from build123d import *

# Parameters (mm, degrees)
BOSS_EXTRUDE1_DEPTH = 60
FILLET1_R           = 5
SKETCH2_R           = 5
CUT_EXTRUDE1_DEPTH  = 75
SKETCH3_W           = 5
SKETCH3_H           = 60
BOSS_EXTRUDE2_DEPTH = 15
FILLET3_R           = 3


with BuildPart() as part:
    # Sketch1 → Boss-Extrude1 (new body)
    with BuildSketch(Plane.XY):
        Polygon((0, 0), (35, 0), (35, -20), (0, -20), (0, -25), (40, -25), (40, 5), (0, 5), align=None)
    extrude(amount=BOSS_EXTRUDE1_DEPTH)

    # Fillet1
    fillet1_edges = [part.edges().sort_by_distance(p)[0] for p in [
        (35, -20, 30),
        (35, 0, 30),
    ]]
    fillet(fillet1_edges, radius=FILLET1_R)

    # Sketch2 → Cut-Extrude1 (cut)
    with BuildSketch(Plane(origin=(0, 5, 0), x_dir=(1, 0, 0), z_dir=(0, 1, 0))):
        with Locations(Location((15, -44, 0), (0, 0, 180))):
            Circle(SKETCH2_R)
        with Locations(Location((15, -16, 0), (0, 0, 270))):
            Circle(SKETCH2_R)
    extrude(amount=-CUT_EXTRUDE1_DEPTH, mode=Mode.SUBTRACT)

    # Sketch3 → Boss-Extrude2 (add)
    with BuildSketch(Plane.XZ.offset(25)):
        with Locations((35, 30)):
            Rectangle(SKETCH3_W, SKETCH3_H)
    extrude(amount=BOSS_EXTRUDE2_DEPTH)

    # Fillet3
    fillet3_edges = [part.edges().sort_by_distance(p)[0] for p in [
        (35, -40, 0),
        (35, -40, 60),
    ]]
    fillet(fillet3_edges, radius=FILLET3_R)


solid = part.part
Build history of the part. All positions in model axes, mm. A direction names the side the tool comes from. Round coordinates to 2 decimals unless told otherwise and drop trailing zeros. Write each loop counter-clockwise with the first axis right and the second up, starting at its lowest first coordinate (ties: lowest second). Pieces come first, ordered by that corner, then holes. Notation, with made-up numbers: M -15,3.5 L 8,3.5 A13 cw 8,9.5 Z; hole C -6.75,45.25 d5. An arc over 180 degrees is marked long. Use CSV: the item, a comma, the result in double quotes.
1. Saw through at A-A (x = 15). Give the cut face in (y, z).
Reply:
outline,"M -25,0 L -20,0 L -20,11 L -25,11 Z; M -25,21 L -20,21 L -20,39 L -25,39 Z; M -25,49 L -20,49 L -20,60 L -25,60 Z; M 0,0 L 5,0 L 5,11 L 0,11 Z; M 0,21 L 5,21 L 5,39 L 0,39 Z; M 0,49 L 5,49 L 5,60 L 0,60 Z"
2. Tool access for faces 1 (the face through (15, 0, 30)), 2 (the face through (39, -25, 30)), 3 (the face through (32.5, -32, 30)), 4 (the face through (15.651, 2.535, 48.957)): list every direction of +Z, -Z, +X, -X, +Y, -Y with a clear straight run to the whole face (end or side of a thin tool).
Reply:
face 1,"+Z, -Z, -X"
face 2,"+Z, -Z, +X, -Y"
face 3,"+Z, -Z, -X, -Y"
face 4,"+Y, -Y"
3. Saw through at D-D (z = 52). Give the cut face in (x, y).
Reply:
outline,"M 0,-25 L 32.5,-25 L 32.5,-40 L 37.5,-40 L 37.5,-25 L 40,-25 L 40,5 L 0,5 L 0,0 L 30,0 A5 cw 35,-5 L 35,-15 A5 cw 30,-20 L 0,-20 Z"
4. Saw through at B-B (z = 19). Give the cut face in (x, y), plus the area to 3 significant figures.
Reply:
outline,"M 0,-25 L 11,-25 L 11,-20 L 0,-20 Z; M 0,0 L 11,0 L 11,5 L 0,5 Z; M 19,-25 L 32.5,-25 L 32.5,-40 L 37.5,-40 L 37.5,-25 L 40,-25 L 40,5 L 19,5 L 19,0 L 30,0 A5 cw 35,-5 L 35,-15 A5 cw 30,-20 L 19,-20 Z"
area,"506 mm²"
5. Wall check: probe 1 along X at (y, z) = (3, 16); probe 2 along Y at (x, z) = (28.5, 40.5); probe 3 along Z at (x, y) = (13, -20.5). Give the ranges that are in metal, low to high. Write a range as from..to.
Reply:
probe 1,"x = 0..10, 20..40"
probe 2,"y = -25..-20, 0..5"
probe 3,"z = 0..11.42, 20.58..39.42, 48.58..60"
6. Flat gauge pins, fed straight in: pin 1 (8 mm diameter, centred on x = 26, z = 44, fed in from -Y); pin 2 (12 mm diameter, centred on y = -33.5, z = 38.5, fed in from +X); pin 3 (4.5 mm diameter, centred on y = -30, z = 37.5, fed in from -X). Where does each tip first touch, or does it go through?
Reply:
pin 1,"stops at y = -25"
pin 2,"stops at x = 37.5"
pin 3,"stops at x = 32.5"
7. Two-plate mould, pull along Y, no slides. Class faces 5 (the face through (33, -1, 30)), 6 (the face through (20, 5, 30)), 7 (the face through (37.5, -32, 30)), 8 (the face through (34, -18, 30)): +Y half, -Y half, draft (parallel to the pull), parting line (faces both ways), or undercut.
Reply:
face 5,"undercut"
face 6,"+Y half"
face 7,"draft"
face 8,"undercut"
8. Saw through at C-C (x = 21.5). Give the cut face in (y, z), plus the area to 3 significant figures.
Reply:
outline,"M -25,0 L -20,0 L -20,60 L -25,60 Z; M 0,0 L 5,0 L 5,60 L 0,60 Z"
area,"600 mm²"
